Here's how the part is built. I have some questions about the finished solid (model axes, mm). Round coordinates to 2 decimals unless told otherwise and drop trailing zeros. Order: outer loops, then holes, each group sorted by start corner. A loop starts at its lowest first (then second) coordinate and runs counter-clockwise, first axis right, second up. Notation, with made-up numbers: (71, 36.5) -> (79, 36.5) arc R31 cw to (79, 65.5) -> close; hole circle Ø10 at (10, -4). An arc over 180 degrees is marked (long way). Use a Markdown table: item, result. Add a question column.
(1) I want a section at C-C, the plane z = 4.2. Please give me the cut outline in (x, y).
(2) I'm going to push a flat-ended pin straight in: P1, Ø6.5, axis at x = -18.5, y = 80, coming from the +Z side. Where does the tip first touch, or does it pass through?
(3) If I drill on probe 1 along Y at (x, z) = (-18, 0.4); probe 2 along Y at (x, z) = (26, 2.4); probe 3 along X at (y, z) = (-109, 0.5), over which ranges is the centre line in solid material (lowest first)?
(4) I want a section at B-B, the plane x = -18.5. Please give me the cut outline in (y, z).
(5) I want a section at A-A, the plane y = -110. Please give me the cut outline in (x, z), then the cut area to 3 significant figures.
(6) I want a section at D-D, the plane x = 0. Please give me the cut outline in (y, z).
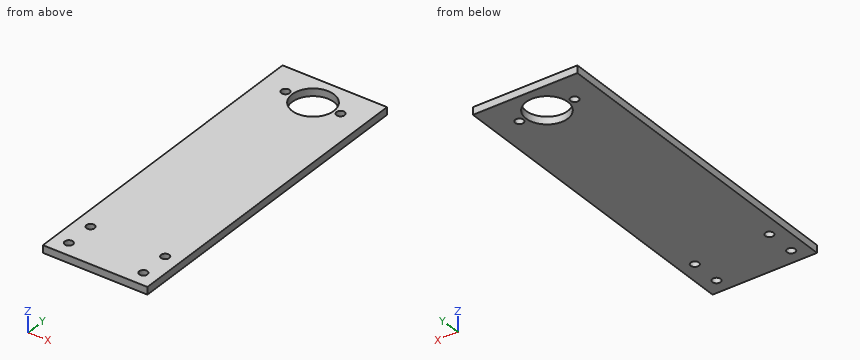
from build123d import *

# Parameters (mm, degrees)
SKETCH1_R           = 14
SKETCH1_R_2         = 2.75
BOSS_EXTRUDE1_DEPTH = 5


with BuildPart() as part:
    # Sketch1 → Boss-Extrude1 (new body)
    with BuildSketch(Plane.XY):
        Polygon((-35, -120), (35, -120), (35, -100), (35, 100), (-35, 100), (-35, -100), align=None)
        with Locations((0, 80)):
            Circle(SKETCH1_R, mode=Mode.SUBTRACT)
        with Locations((-25, -110)):
            Circle(SKETCH1_R_2, mode=Mode.SUBTRACT)
        with Locations((25, -110)):
            Circle(SKETCH1_R_2, mode=Mode.SUBTRACT)
        with Locations((25, -90)):
            Circle(SKETCH1_R_2, mode=Mode.SUBTRACT)
        with Locations((-25, -90)):
            Circle(SKETCH1_R_2, mode=Mode.SUBTRACT)
        with Locations((18.5, 80)):
            Circle(SKETCH1_R_2, mode=Mode.SUBTRACT)
        with Locations((-18.5, 80)):
            Circle(SKETCH1_R_2, mode=Mode.SUBTRACT)
    extrude(amount=BOSS_EXTRUDE1_DEPTH)


solid = part.part
Taken from the geometry:
| question | item | result |
|---|---|---|
| 1 | outline | (-35, -120) -> (35, -120) -> (35, 100) -> (-35, 100) -> close; hole circle Ø5.5 at (-25, -110); hole circle Ø5.5 at (-25, -90); hole circle Ø5.5 at (-18.5, 80); hole circle Ø28 at (0, 80); hole circle Ø5.5 at (18.5, 80); hole circle Ø5.5 at (25, -110); hole circle Ø5.5 at (25, -90) |
| 2 | P1 | stops at z = 5 |
| 3 | probe 1 | y = -120 to 77.3, 82.7 to 100 |
| 3 | probe 2 | y = -120 to -112.56, -107.44 to -92.56, -87.44 to 100 |
| 3 | probe 3 | x = -35 to -27.56, -22.44 to 22.44, 27.56 to 35 |
| 4 | outline | (-120, 0) -> (77.25, 0) -> (77.25, 5) -> (-120, 5) -> close; (82.75, 0) -> (100, 0) -> (100, 5) -> (82.75, 5) -> close |
| 5 | outline | (-35, 0) -> (-27.75, 0) -> (-27.75, 5) -> (-35, 5) -> close; (-22.25, 0) -> (22.25, 0) -> (22.25, 5) -> (-22.25, 5) -> close; (27.75, 0) -> (35, 0) -> (35, 5) -> (27.75, 5) -> close |
| 5 | area | 295 mm2 |
| 6 | outline | (-120, 0) -> (66, 0) -> (66, 5) -> (-120, 5) -> close; (94, 0) -> (100, 0) -> (100, 5) -> (94, 5) -> close |
